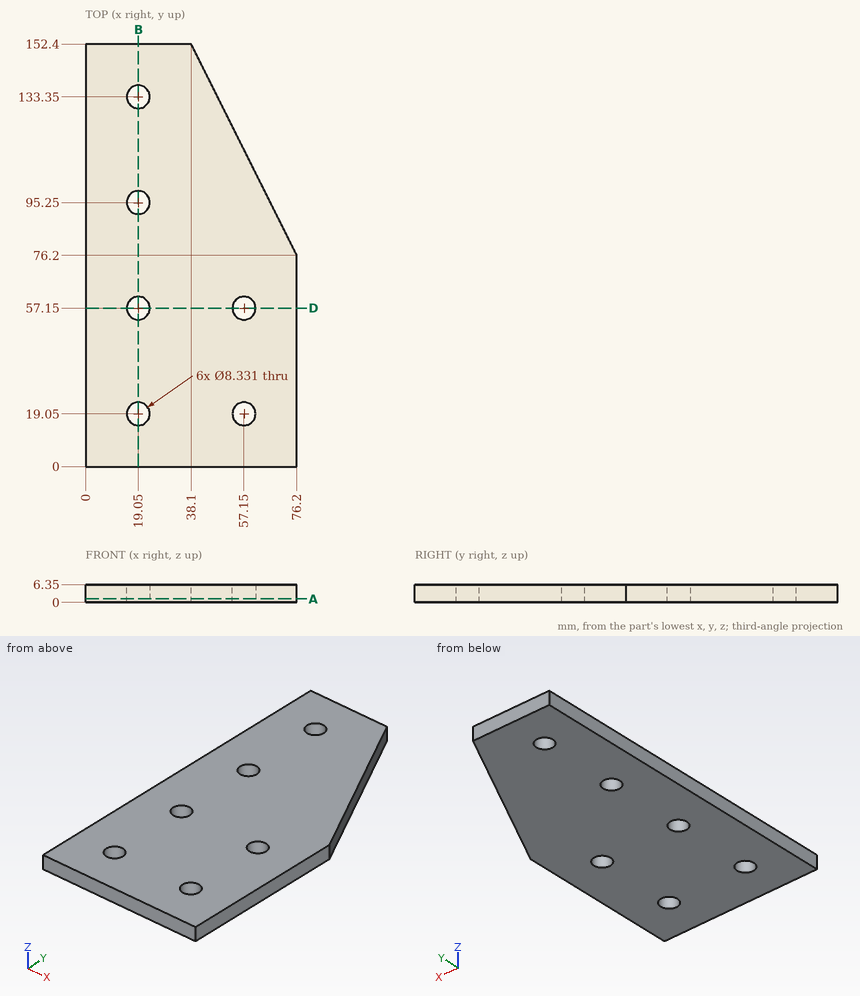
The drawing under review shows one solid part. Ordinate dimensions are in mm from its lowest x, y, z. Round coordinates to 2 decimals unless told otherwise and drop trailing zeros. Loops run counter-clockwise (first coordinate to the right, second up) from the corner with the lowest first, then second, coordinate; pieces in that order, holes last.
Item 1: Take a section at A-A (z = 1.25). Write out the cut boundary in (x, y), then the cut area to 3 significant figures.
Determined:
outline: (0, 0) - (76.2, 0) - (76.2, 76.2) - (38.1, 152.4) - (0, 152.4) - close; hole circle Ø8.33 at (19.05, 19.05); hole circle Ø8.33 at (19.05, 57.15); hole circle Ø8.33 at (19.05, 95.25); hole circle Ø8.33 at (19.05, 133.35); hole circle Ø8.33 at (57.15, 19.05); hole circle Ø8.33 at (57.15, 57.15)
area: 9,830 mm2
Item 2: Take a section at D-D (y = 57.15). Write out the cut boundary in (x, z), then the cut area to 3 significant figures.
Determined:
outline: (0, 0) - (14.88, 0) - (14.88, 6.35) - (0, 6.35) - close; (23.22, 0) - (52.98, 0) - (52.98, 6.35) - (23.22, 6.35) - close; (61.32, 0) - (76.2, 0) - (76.2, 6.35) - (61.32, 6.35) - close
area: 378 mm2
Item 3: Take a section at B-B (x = 19.05). Write out the cut boundary in (y, z).
Determined:
outline: (0, 0) - (14.88, 0) - (14.88, 6.35) - (0, 6.35) - close; (23.22, 0) - (52.98, 0) - (52.98, 6.35) - (23.22, 6.35) - close; (61.32, 0) - (91.08, 0) - (91.08, 6.35) - (61.32, 6.35) - close; (99.42, 0) - (129.18, 0) - (129.18, 6.35) - (99.42, 6.35) - close; (137.52, 0) - (152.4, 0) - (152.4, 6.35) - (137.52, 6.35) - close
Item 4: For line 1 (Y direction, x = 19.05, z = 4); line 2 (X direction, y = 21, z = 0.5); line 3 (X direction, y = 21.5, z = 3), list the stretches that pass through material, from the lowest coordinate up.
Determined:
line 1: y = 0 to 14.88, 23.22 to 52.98, 61.32 to 91.08, 99.42 to 129.18, 137.52 to 152.4
line 2: x = 0 to 15.37, 22.73 to 53.47, 60.83 to 76.2
line 3: x = 0 to 15.68, 22.42 to 53.78, 60.52 to 76.2
